from build123d import *

# Parameters (mm, degrees)
F1_DEPTH = 101.6
F0_W     = 25.4
F0_H     = 19.05
F2_DEPTH = 25.4
F3_DEPTH = 7.9375
F5_R     = 6.35
F6_R     = 6.35
F7_DEPTH = 19.051


# Not quite as in the source:
# - a feature names something its author has since deleted; it is built from what else it names


with BuildPart() as f1:
    # F0 (on Front) → F1 (new body, symmetric)
    with BuildSketch(Plane.XZ):
        Polygon((-92.075, -9.525), (-41.275, -9.525), (41.275, -9.525), (92.075, -9.525), (92.075, 9.525), (41.275, 9.525), (22.225, 9.525), (-41.275, 9.525), (-92.075, 9.525), align=None)
    extrude(amount=F1_DEPTH, both=True)

    # F0 (on Front) → F2 (join, symmetric)
    with BuildSketch(Plane.XZ):
        with BuildLine():
            Line((22.225, 9.525), (41.275, 9.525))
            Line((41.275, 9.525), (41.275, 27.0002))
            ThreePointArc((41.275, 27.0002), (45.9246798487, 38.2255201513), (57.15, 42.8752))
            Line((57.15, 42.8752), (60.325, 42.8752))
            Line((60.325, 42.8752), (60.325, 61.9252))
            Line((60.325, 61.9252), (57.15, 61.9252))
            ThreePointArc((57.15, 61.9252), (32.4542956671, 51.6959043329), (22.225, 27.0002))
            Line((22.225, 27.0002), (22.225, 9.525))
        make_face()
        with Locations((73.025, 52.4002)):
            Rectangle(F0_W, F0_H)
    extrude(amount=F2_DEPTH, both=True)

    # F0 (on Front) → F3 (join, symmetric)
    with BuildSketch(Plane.XZ):
        with BuildLine():
            add(Edge.make_bspline(
                [(-41.275, 9.525), (-41.1597527564, 29.4812973589), (32.6236560941, 62.2739233077), (57.15, 61.9252)],
                knots=[0, 0, 0, 0, 111.5045361635, 111.5045361635, 111.5045361635, 111.5045361635], degree=3))
            Line((-41.275, 9.525), (22.225, 9.525))
            Line((22.225, 9.525), (22.225, 27.0002))
            ThreePointArc((22.225, 27.0002), (32.4542956671, 51.6959043329), (57.15, 61.9252))
        make_face()
    extrude(amount=F3_DEPTH, both=True)

    # F0 (on Front) → F4 (revolve)
    with BuildSketch(Plane.XZ):
        Polygon((85.725, 66.675), (85.725, 61.9252), (85.725, 42.8752), (85.725, 38.1), (111.125, 38.1), (111.125, 66.675), align=None)
    revolve(axis=Axis((85.725, 0, 52.3875), (0, 0, 1)))

    # F5
    f5_edges = [f1.edges().sort_by_distance(p)[0] for p in [
        (-92.075, -101.6, 0),
        (92.075, -101.6, 0),
        (92.075, 101.6, 0),
        (-92.075, 101.6, 0),
    ]]
    fillet(f5_edges, radius=F5_R)

    # F6 (on face) → F7 (cut, through all)
    with BuildSketch(Plane.XY.offset(9.525)):
        with Locations((66.675, 76.2)):
            Circle(F6_R)
        with Locations((66.675, -76.2)):
            Circle(F6_R)
        with Locations((-66.675, 76.2)):
            Circle(F6_R)
        with Locations((-66.675, -76.2)):
            Circle(F6_R)
    extrude(amount=-F7_DEPTH, mode=Mode.SUBTRACT)


solid = f1.part
Read the model definition and answer for the solid it produces. Units are mm, in the model's axes. A direction names the side the tool comes from. Round coordinates to 2 decimals unless told otherwise and drop trailing zeros. Loops run counter-clockwise (first coordinate to the right, second up) from the corner with the lowest first, then second, coordinate; pieces in that order, holes last.
Q1. Section A-A on y = 76.2 is taken. Write down the section's boundary in (x, z) (3 decimals).
Q2. Consider probe 1 along X at (y, z) = (76, 2) (3 decimals); probe 2 along Y at (x, z) = (-67.5, -1); probe 3 along Z at (x, y) = (78.5, 30) (3 decimals). Determine where each line is inside the solid, lowest interval first.
Q3. Section B-B on z = 1.5 is taken. Write down the section's boundary in (x, y) (3 decimals).
Q4. Section C-C on y = -51.5 is taken. Write down the section's boundary in (x, z) (3 decimals), and give its area (3 significant figures).
Q5. Which of the six approach directions +Z, -Z, +X, -X, +Y, -Y give full straight-line access (tool end or side, diameter ignored) to faces 5 (the face through (60, -2, 61.925)), 6 (the face through (-2, -7.938, 25)), 7 (the face through (46, 25.4, 42)), 8 (the face through (92.075, -1, 0)), 9 (the face through (-2, 7.938, 25))?
Q6. Determine the mould class of faces 1 (the face through (-1, -1, -9.525)), 2 (the face through (41.275, 0, 18)), 3 (the face through (-90.165, 99.789, -0.133)), 4 (the face through (86, 0, 38.1)) for opening direction Z: released by +Z, released by -Z, zero draft, split by the parting line, or undercut.
Q7. Each of these flat-tipped pins is pushed along its axis until it touches: pin 1 (15.5 mm diameter, centred on x = -5, z = 29.5, fed in from +Y); pin 2 (20.5 mm diameter, centred on x = -66.675, y = 76.2, fed in from +Z) (3 decimals); pin 3 (15 mm diameter, centred on y = 0, z = 3, fed in from +X) (3 decimals). Where does it stop, or does it pass through?
Output:
1. outline: (-92.075, -9.525) - (-73.025, -9.525) - (-73.025, 9.525) - (-92.075, 9.525) - close; (-60.325, -9.525) - (60.325, -9.525) - (60.325, 9.525) - (-60.325, 9.525) - close; (73.025, -9.525) - (92.075, -9.525) - (92.075, 9.525) - (73.025, 9.525) - close
2. probe 1: x = -92.075 to -73.022, -60.328 to 60.328, 73.022 to 92.075
2. probe 2: y = -101.6 to -82.5, -69.9 to 69.9, 82.5 to 101.6
2. probe 3: z = -9.525 to 9.525
3. outline: (-92.075, -95.25) arc R6.35 ccw to (-85.725, -101.6) - (85.725, -101.6) arc R6.35 ccw to (92.075, -95.25) - (92.075, 95.25) arc R6.35 ccw to (85.725, 101.6) - (-85.725, 101.6) arc R6.35 ccw to (-92.075, 95.25) - close; hole circle Ø12.7 at (-66.675, -76.2); hole circle Ø12.7 at (-66.675, 76.2); hole circle Ø12.7 at (66.675, -76.2); hole circle Ø12.7 at (66.675, 76.2)
4. outline: (-92.075, -9.525) - (92.075, -9.525) - (92.075, 9.525) - (-92.075, 9.525) - close
4. area: 3,510 mm2
5. face 5: +Z, -X
5. face 6: +Z, -X, -Y
5. face 7: +Z, +X, -X, +Y
5. face 8: -Z, +X, +Y, -Y
5. face 9: +Z, -X, +Y
6. face 1: released by -Z
6. face 2: undercut
6. face 3: zero draft
6. face 4: undercut
7. pin 1: stops at y = 7.94
7. pin 2: stops at z = 9.525
7. pin 3: stops at x = 92.075
